Could you check a few things on this drawing? It's one solid part, dimensions in mm from its lowest x, y, z. A direction names the side the tool comes from. Coordinates: 2 decimals unless noted, no trailing zeros. Loops run counter-clockwise (first coordinate to the right, second up) from the corner with the lowest first, then second, coordinate; pieces in that order, holes last. Notation, with made-up numbers: M 47,25 L 71,25 A21 ccw 71,36 Z; hole C 72.5,-33.75 d5. An arc over 180 degrees is marked long. Use one line per item in the form item = value. Start each with the question number.
(1) Imagine slicing it at C-C, the plane z = 4.25. Please give me the cut outline in (x, y).
(2) Thinking about a two-plate mould opening in X: for the marked faces 3, 4, 5 and 6, which applies, +X half, -X half, draft (parallel to the pull), parting line (faces both ways), or undercut?
(3) On a 3-axis mill with a long thin cutter (end or side, diameter ignored), from which of +Z, -Z, +X, -X, +Y, -Y can I reach the whole of each face in a straight line? I mean the marked faces 1 and 2. Say none if no direction works.
(4) Imagine slicing it at A-A, the plane x = 42. Please give me the cut outline in (y, z).
(5) Please list where these lines run through material, in increasing order: L1, parallel to Y at x = 57.5, z = 6.5; L2, parallel to Y at x = 93, z = 5.75.
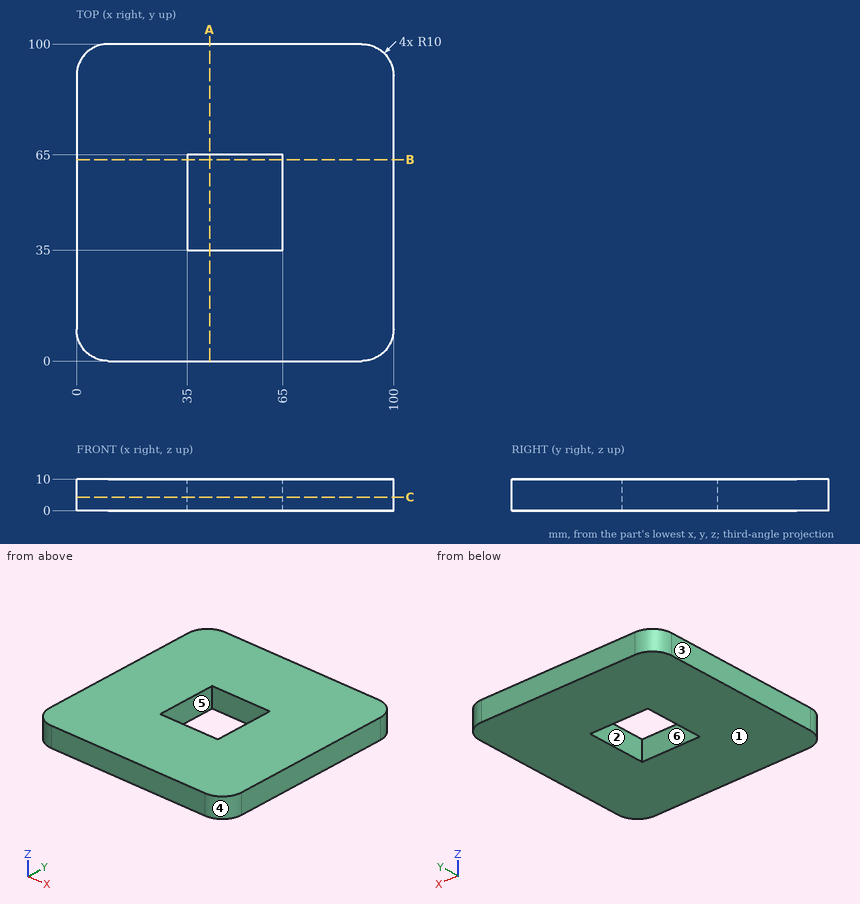
Answer:
q1.outline = M 0,10 A10 ccw 10,0 L 90,0 A10 ccw 100,10 L 100,90 A10 ccw 90,100 L 10,100 A10 ccw 0,90 Z; hole M 35,35 L 65,35 L 65,65 L 35,65 Z
q2.face_3 = -X half
q2.face_4 = +X half
q2.face_5 = undercut
q2.face_6 = undercut
q3.face_1 = -Z, +X, -X, +Y, -Y
q3.face_2 = +Z, -Z
q4.outline = M 0,0 L 35,0 L 35,10 L 0,10 Z; M 65,0 L 100,0 L 100,10 L 65,10 Z
q5.L1 = 0 to 35, 65 to 100
q5.L2 = 0.46 to 99.54
